Can you work these out from the drawing? Everything is in mm from the part's minimum corner. A direction names the side the tool comes from. Coordinates: 2 decimals unless noted, no trailing zeros. Loops run counter-clockwise (first coordinate to the right, second up) from the corner with the lowest first, then second, coordinate; pieces in that order, holes last.
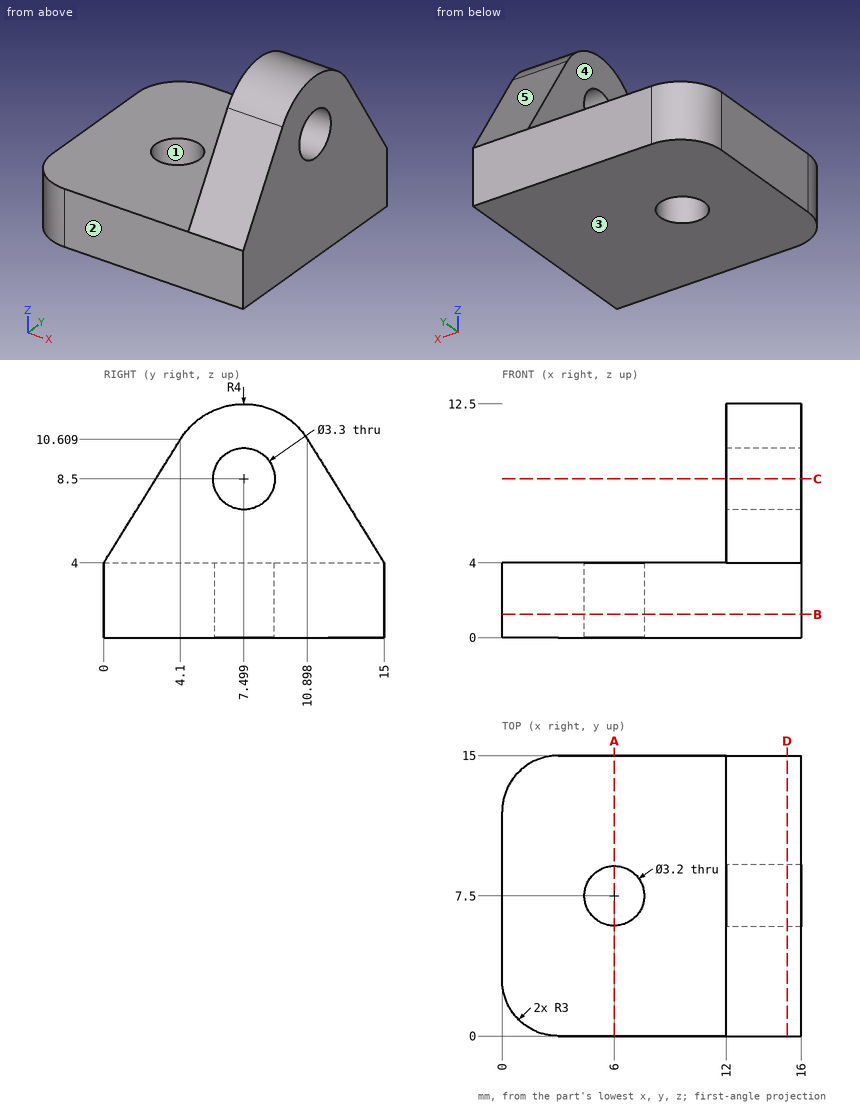
Item 1: I need wall thicknesses on line 1 along Y through (x, z) = (6, 2.4); line 2 along Z through (x, y) = (11.5, 5.5); line 3 along X through (y, z) = (6.75, 5). Which ranges of each line are inside material? Lowest first, please.
Results are:
line 1: y = 0 to 5.9, 9.1 to 15
line 2: z = 0 to 4
line 3: x = 12 to 16
Item 2: Suppose I cut it at B-B, the plane z = 1.25. Please give me the cut outline in (x, y), plus the area to 3 significant figures.
Results are:
outline: (0, 3) arc R3 ccw to (3, 0) - (16, 0) - (16, 15) - (3, 15) arc R3 ccw to (0, 12) - close; hole circle Ø3.2 at (6, 7.5)
area: 228 mm2
Item 3: Suppose I cut it at A-A, the plane x = 6. Please give me the cut outline in (y, z).
Results are:
outline: (0, 0) - (5.9, 0) - (5.9, 4) - (0, 4) - close; (9.1, 0) - (15, 0) - (15, 4) - (9.1, 4) - close
Item 4: On a 3-axis mill with a long thin cutter (end or side, diameter ignored), from which of +Z, -Z, +X, -X, +Y, -Y can I reach the whole of each face in a straight line? I mean the marked faces 4 and 5. Say none if no direction works.
Results are:
face 4: +Z, -X, +Y, -Y
face 5: +Z, +X, -X, +Y
Item 5: Suppose I cut it at C-C, the plane z = 8.5. Please give me the cut outline in (x, y).
Results are:
outline: (12, 2.79) - (16, 2.79) - (16, 5.85) - (12, 5.85) - close; (12, 9.15) - (16, 9.15) - (16, 12.21) - (12, 12.21) - close
Item 6: We'd pull the mould along Y, two halves only. Please class the marked faces 1, 2 and 3: +Y half, -Y half, draft (parallel to the pull), parting line (faces both ways), or undercut.
Results are:
face 1: undercut
face 2: -Y half
face 3: draft
Item 7: Suppose I cut it at D-D, the plane x = 15.25. Please give me the cut outline in (y, z), plus the area to 3 significant figures.
Results are:
outline: (0, 0) - (15, 0) - (15, 4) - (10.9, 10.61) arc R4 ccw to (4.1, 10.61) - (0, 4) - close; hole circle Ø3.3 at (7.5, 8.5)
area: 133 mm2
Item 8: I'm going to push flat-ended pins straight in: P1, Ø1, axis at y = 13, z = 7, coming from the -X side; P2, Ø4, axis at x = 8.5, y = 2, coming from the +Z side; P3, Ø5, axis at x = 12.5, y = 11.5, coming from the +Z side. Where does each tip first touch, or does it pass through?
Results are:
P1: stops at x = 12
P2: stops at z = 4
P3: stops at z = 12.21
